Part model, mm, in its own coordinate system. A direction names the side the tool comes from. Coordinates: 2 decimals unless noted, no trailing zeros. Write each loop counter-clockwise with the first axis right and the second up, starting at its lowest first coordinate (ties: lowest second). Pieces come first, ordered by that corner, then holes. Notation, with made-up numbers: M -4,47 L 21,47 A7 ccw 21,52 Z; hole C 17,-8 d4. An arc over 180 degrees is marked long. Use a Markdown table: item, result. Add a question column.
Q1. Slice it at A-A on x = -37. Write the cut outline in (y, z), then the cut area to 3 significant figures.
Q2. Slice it at D-D on y = 30. Write the cut outline in (x, z).
Q3. Slice it at B-B on y = 0. Write the cut outline in (x, z), then the cut area to 3 significant figures.
Q4. Pin check, flat tip, straight feed: pin 1 Ø3 at (x, z) = (33, 3.5) entering from -Y. Stop position of the tip, or through.
Q5. Tool access for faces 1 (the cylindrical face through (-18.442, 76.791, 3.131)), 2 (the cylindrical face through (57.282, 54.367, 3.131)), 3 (the cylindrical face through (-60.06, 51.29, 3.13)): list every direction of +Z, -Z, +X, -X, +Y, -Y with a clear straight run to the whole face (end or side of a thin tool).
Q6. Slice it at C-C on z = 4. Count the separate pieces of the cut face and the enclosed holes in it, then the cut area to 3 significant figures.
Q7. Mould opens along Y. For faces 4 (the cylindrical face through (2.034, 79.066, 3.131)), 5 (the cylindrical face through (-2.034, -79.066, 3.131)), 6 (the cylindrical face through (-69.946, -0.104, 3.131)) say: released by +Y, released by -Y, zero draft, split by the parting line, or undercut.
Q8. Wall check: L1, parallel to Y at x = 16, z = 1.5; L2, parallel to Y at x = 57, z = 1; L3, parallel to Y at x = -37, z = 5. Give the ranges that are in metal, low to high. Write a range as from..to.
from build123d import *

# Parameters (mm, degrees)
BOSS_EXTRUDE1_DEPTH = 6.35
SKETCH2_R           = 3.96875
CUT_EXTRUDE1_DEPTH  = 118.165311767


with BuildPart() as part:
    # Sketch1 → Boss-Extrude1 (new body)
    with BuildSketch(Plane.XY):
        with BuildLine():
            ThreePointArc((-2.76225, 74.614024644), (-2.053719894, 79.00655424), (0, 82.953523426))
            ThreePointArc((0, 82.953523426), (2.053719894, 79.00655424), (2.76225, 74.614024644))
            ThreePointArc((2.76225, 74.614024644), (7.311245407, 69.561853415), (12.811239812, 73.557833254))
            ThreePointArc((12.811239812, 73.557833254), (14.417545091, 77.707063847), (17.247007315, 81.140789912))
            ThreePointArc((17.247007315, 81.140789912), (18.435227465, 76.853079096), (18.215016233, 72.409225119))
            ThreePointArc((18.215016233, 72.409225119), (21.614199713, 66.521666626), (27.82481697, 69.286811582))
            ThreePointArc((27.82481697, 69.286811582), (30.258694172, 73.011401885), (33.74023765, 75.781814521))
            ThreePointArc((33.74023765, 75.781814521), (34.011027133, 71.340755614), (32.87169885, 67.039794998))
            ThreePointArc((32.87169885, 67.039794998), (34.972509775, 60.574163799), (41.622316107, 61.987623769))
            ThreePointArc((41.622316107, 61.987623769), (44.777393121, 65.124791313), (48.758857695, 67.110810195))
            ThreePointArc((48.758857695, 67.110810195), (48.100381712, 62.710498781), (46.091730493, 58.740404142))
            ThreePointArc((46.091730493, 58.740404142), (46.802353344, 51.979279347), (53.600720305, 51.979279347))
            ThreePointArc((53.600720305, 51.979279347), (57.339105124, 54.391914857), (61.646481689, 55.50674143))
            ThreePointArc((61.646481689, 55.50674143), (60.0875188, 51.339492232), (57.29733234, 47.873775759))
            ThreePointArc((57.29733234, 47.873775759), (56.586709488, 41.112650963), (63.23651582, 39.699190994))
            ThreePointArc((63.23651582, 39.699190994), (67.39482309, 41.28185072), (71.83985862, 41.476761713))
            ThreePointArc((71.83985862, 41.476761713), (69.448542984, 37.724703519), (65.99876582, 34.91483365))
            ThreePointArc((65.99876582, 34.91483365), (63.897954895, 28.449202452), (70.108572152, 25.684057496))
            ThreePointArc((70.108572152, 25.684057496), (74.505063891, 26.367571615), (78.893489004, 25.634048482))
            ThreePointArc((78.893489004, 25.634048482), (75.774332589, 22.461164239), (71.815736537, 20.429945772))
            ThreePointArc((71.815736537, 20.429945772), (68.416553057, 14.542387279), (73.916547462, 10.54640744))
            ThreePointArc((73.916547462, 10.54640744), (78.359075884, 10.300903104), (82.499095345, 8.671004326))
            ThreePointArc((82.499095345, 8.671004326), (78.788420253, 6.215964301), (74.494014958, 5.052171229))
            ThreePointArc((74.494014958, 5.052171229), (69.945019551, 0), (74.494014958, -5.052171229))
            ThreePointArc((74.494014958, -5.052171229), (78.788420253, -6.215964301), (82.499095345, -8.671004326))
            ThreePointArc((82.499095345, -8.671004326), (78.359075884, -10.300903104), (73.916547462, -10.54640744))
            ThreePointArc((73.916547462, -10.54640744), (68.416553057, -14.542387279), (71.815736537, -20.429945772))
            ThreePointArc((71.815736537, -20.429945772), (75.774332589, -22.461164239), (78.893489004, -25.634048482))
            ThreePointArc((78.893489004, -25.634048482), (74.505063891, -26.367571615), (70.108572152, -25.684057496))
            ThreePointArc((70.108572152, -25.684057496), (63.897954895, -28.449202452), (65.99876582, -34.91483365))
            ThreePointArc((65.99876582, -34.91483365), (69.448542984, -37.724703519), (71.83985862, -41.476761713))
            ThreePointArc((71.83985862, -41.476761713), (67.39482309, -41.28185072), (63.23651582, -39.699190994))
            ThreePointArc((63.23651582, -39.699190994), (56.586709488, -41.112650963), (57.29733234, -47.873775759))
            ThreePointArc((57.29733234, -47.873775759), (60.0875188, -51.339492232), (61.646481689, -55.50674143))
            ThreePointArc((61.646481689, -55.50674143), (57.339105124, -54.391914857), (53.600720305, -51.979279347))
            ThreePointArc((53.600720305, -51.979279347), (46.802353344, -51.979279347), (46.091730493, -58.740404142))
            ThreePointArc((46.091730493, -58.740404142), (48.100381712, -62.710498781), (48.758857695, -67.110810195))
            ThreePointArc((48.758857695, -67.110810195), (44.777393121, -65.124791313), (41.622316107, -61.987623769))
            ThreePointArc((41.622316107, -61.987623769), (34.972509775, -60.574163799), (32.87169885, -67.039794998))
            ThreePointArc((32.87169885, -67.039794998), (34.011027133, -71.340755614), (33.74023765, -75.781814521))
            ThreePointArc((33.74023765, -75.781814521), (30.258694172, -73.011401885), (27.82481697, -69.286811582))
            ThreePointArc((27.82481697, -69.286811582), (21.614199713, -66.521666626), (18.215016233, -72.409225119))
            ThreePointArc((18.215016233, -72.409225119), (18.435227465, -76.853079096), (17.247007315, -81.140789912))
            ThreePointArc((17.247007315, -81.140789912), (14.417545091, -77.707063847), (12.811239812, -73.557833254))
            ThreePointArc((12.811239812, -73.557833254), (7.311245407, -69.561853415), (2.76225, -74.614024644))
            ThreePointArc((2.76225, -74.614024644), (2.053719894, -79.00655424), (0, -82.953523426))
            ThreePointArc((0, -82.953523426), (-2.053719894, -79.00655424), (-2.76225, -74.614024644))
            ThreePointArc((-2.76225, -74.614024644), (-7.311245407, -69.561853415), (-12.811239812, -73.557833254))
            ThreePointArc((-12.811239812, -73.557833254), (-14.417545091, -77.707063847), (-17.247007315, -81.140789912))
            ThreePointArc((-17.247007315, -81.140789912), (-18.435227465, -76.853079096), (-18.215016233, -72.409225119))
            ThreePointArc((-18.215016233, -72.409225119), (-21.614199713, -66.521666626), (-27.82481697, -69.286811582))
            ThreePointArc((-27.82481697, -69.286811582), (-30.258694172, -73.011401885), (-33.74023765, -75.781814521))
            ThreePointArc((-33.74023765, -75.781814521), (-34.011027133, -71.340755614), (-32.87169885, -67.039794998))
            ThreePointArc((-32.87169885, -67.039794998), (-34.972509775, -60.574163799), (-41.622316107, -61.987623769))
            ThreePointArc((-41.622316107, -61.987623769), (-44.777393121, -65.124791313), (-48.758857695, -67.110810195))
            ThreePointArc((-48.758857695, -67.110810195), (-48.100381712, -62.710498781), (-46.091730493, -58.740404142))
            ThreePointArc((-46.091730493, -58.740404142), (-46.802353344, -51.979279347), (-53.600720305, -51.979279347))
            ThreePointArc((-53.600720305, -51.979279347), (-57.339105124, -54.391914857), (-61.646481689, -55.50674143))
            ThreePointArc((-61.646481689, -55.50674143), (-60.0875188, -51.339492232), (-57.29733234, -47.873775759))
            ThreePointArc((-57.29733234, -47.873775759), (-56.586709488, -41.112650963), (-63.23651582, -39.699190994))
            ThreePointArc((-63.23651582, -39.699190994), (-67.39482309, -41.28185072), (-71.83985862, -41.476761713))
            ThreePointArc((-71.83985862, -41.476761713), (-69.448542984, -37.724703519), (-65.99876582, -34.91483365))
            ThreePointArc((-65.99876582, -34.91483365), (-63.897954895, -28.449202452), (-70.108572152, -25.684057496))
            ThreePointArc((-70.108572152, -25.684057496), (-74.505063891, -26.367571615), (-78.893489004, -25.634048482))
            ThreePointArc((-78.893489004, -25.634048482), (-75.774332589, -22.461164239), (-71.815736537, -20.429945772))
            ThreePointArc((-71.815736537, -20.429945772), (-68.416553057, -14.542387279), (-73.916547462, -10.54640744))
            ThreePointArc((-73.916547462, -10.54640744), (-78.359075884, -10.300903104), (-82.499095345, -8.671004326))
            ThreePointArc((-82.499095345, -8.671004326), (-78.788420253, -6.215964301), (-74.494014958, -5.052171229))
            ThreePointArc((-74.494014958, -5.052171229), (-69.945019551, 0), (-74.494014958, 5.052171229))
            ThreePointArc((-74.494014958, 5.052171229), (-78.788420253, 6.215964301), (-82.499095345, 8.671004326))
            ThreePointArc((-82.499095345, 8.671004326), (-78.359075884, 10.300903104), (-73.916547462, 10.54640744))
            ThreePointArc((-73.916547462, 10.54640744), (-68.416553057, 14.542387279), (-71.815736537, 20.429945772))
            ThreePointArc((-71.815736537, 20.429945772), (-75.774332589, 22.461164239), (-78.893489004, 25.634048482))
            ThreePointArc((-78.893489004, 25.634048482), (-74.505063891, 26.367571615), (-70.108572152, 25.684057496))
            ThreePointArc((-70.108572152, 25.684057496), (-63.897954895, 28.449202452), (-65.99876582, 34.91483365))
            ThreePointArc((-65.99876582, 34.91483365), (-69.448542984, 37.724703519), (-71.83985862, 41.476761713))
            ThreePointArc((-71.83985862, 41.476761713), (-67.39482309, 41.28185072), (-63.23651582, 39.699190994))
            ThreePointArc((-63.23651582, 39.699190994), (-56.586709488, 41.112650963), (-57.29733234, 47.873775759))
            ThreePointArc((-57.29733234, 47.873775759), (-60.0875188, 51.339492232), (-61.646481689, 55.50674143))
            ThreePointArc((-61.646481689, 55.50674143), (-57.339105124, 54.391914857), (-53.600720305, 51.979279347))
            ThreePointArc((-53.600720305, 51.979279347), (-46.802353344, 51.979279347), (-46.091730493, 58.740404142))
            ThreePointArc((-46.091730493, 58.740404142), (-48.100381712, 62.710498781), (-48.758857695, 67.110810195))
            ThreePointArc((-48.758857695, 67.110810195), (-44.777393121, 65.124791313), (-41.622316107, 61.987623769))
            ThreePointArc((-41.622316107, 61.987623769), (-34.972509775, 60.574163799), (-32.87169885, 67.039794998))
            ThreePointArc((-32.87169885, 67.039794998), (-34.011027133, 71.340755614), (-33.74023765, 75.781814521))
            ThreePointArc((-33.74023765, 75.781814521), (-30.258694172, 73.011401885), (-27.82481697, 69.286811582))
            ThreePointArc((-27.82481697, 69.286811582), (-21.614199713, 66.521666626), (-18.215016233, 72.409225119))
            ThreePointArc((-18.215016233, 72.409225119), (-18.435227465, 76.853079096), (-17.247007315, 81.140789912))
            ThreePointArc((-17.247007315, 81.140789912), (-14.417545091, 77.707063847), (-12.811239812, 73.557833254))
            ThreePointArc((-12.811239812, 73.557833254), (-7.311245407, 69.561853415), (-2.76225, 74.614024644))
        make_face()
    extrude(amount=BOSS_EXTRUDE1_DEPTH)

    # Sketch2 → Cut-Extrude1 (cut, through all)
    with BuildSketch(Plane.XY.offset(6.35)):
        with Locations((-37, 0)):
            Circle(SKETCH2_R)
        with Locations((-18.5, 32.04293994)):
            Circle(SKETCH2_R)
        with Locations((18.5, 32.04293994)):
            Circle(SKETCH2_R)
        with Locations((37, 0)):
            Circle(SKETCH2_R)
        with Locations((18.5, -32.04293994)):
            Circle(SKETCH2_R)
        with Locations((-18.5, -32.04293994)):
            Circle(SKETCH2_R)
        with BuildLine():
            ThreePointArc((-11.27698735, 14.154471469), (-15.672894745, 9.04875), (-17.896625544, 2.688921789))
            ThreePointArc((-17.896625544, 2.688921789), (-28.728141104, -16.5862), (-6.619638194, -16.843393258))
            ThreePointArc((-6.619638194, -16.843393258), (0, -18.0975), (6.619638194, -16.843393258))
            ThreePointArc((6.619638194, -16.843393258), (28.728141104, -16.5862), (17.896625544, 2.688921789))
            ThreePointArc((17.896625544, 2.688921789), (15.672894745, 9.04875), (11.27698735, 14.154471469))
            ThreePointArc((11.27698735, 14.154471469), (0, 33.1724), (-11.27698735, 14.154471469))
        make_face()
    extrude(amount=-CUT_EXTRUDE1_DEPTH, mode=Mode.SUBTRACT)


solid = part.part
Recorded:
| question | item | result |
|---|---|---|
| 1 | outline | M -59.92,0 L -3.97,0 L -3.97,6.35 L -59.92,6.35 Z; M 3.97,0 L 59.92,0 L 59.92,6.35 L 3.97,6.35 Z |
| 1 | area | 711 mm² |
| 2 | outline | M -63.48,0 L -21.9,0 L -21.9,6.35 L -63.48,6.35 Z; M -15.1,0 L -8.45,0 L -8.45,6.35 L -15.1,6.35 Z; M 8.45,0 L 15.1,0 L 15.1,6.35 L 8.45,6.35 Z; M 21.9,0 L 63.48,0 L 63.48,6.35 L 21.9,6.35 Z |
| 3 | outline | M -69.95,0 L -40.97,0 L -40.97,6.35 L -69.95,6.35 Z; M -33.03,0 L -25.47,0 L -25.47,6.35 L -33.03,6.35 Z; M 25.47,0 L 33.03,0 L 33.03,6.35 L 25.47,6.35 Z; M 40.97,0 L 69.95,0 L 69.95,6.35 L 40.97,6.35 Z |
| 3 | area | 464 mm² |
| 4 | pin 1 | y = -75.78 |
| 5 | face 1 | +Z, -Z |
| 5 | face 2 | +Z, -Z, +Y |
| 5 | face 3 | +Z, -Z, -X |
| 6 | separate pieces | 1 |
| 6 | enclosed holes | 7 |
| 6 | area | 15,000 mm² |
| 7 | face 4 | released by +Y |
| 7 | face 5 | released by -Y |
| 7 | face 6 | undercut |
| 8 | L1 | -79.9..-35.13, -28.96..-22.91, 8.46..28.96, 35.13..79.9 |
| 8 | L2 | -54.24..-47.58, -40.61..40.61, 47.58..54.24 |
| 8 | L3 | -59.92..-3.97, 3.97..59.92 |
